For this review, take the finished solid that the model builds, in its own axes (mm). A direction names the side the tool comes from. Give positions to 0.01 mm unless a question says otherwise; leave off trailing zeros. Order: outer loops, then holes, each group sorted by start corner. A loop starts at its lowest first (then second) coordinate and runs counter-clockwise, first axis right, second up. Notation, with made-up numbers: M 65,36.25 L 75,36.25 A24 ccw 75,57.25 Z; hole C 82.25,70.5 d8. An arc over 180 degrees is marked long. Use CSV: the item, a comma, the result in double quotes. Start each with the question number.
(1) Consider section A-A (y = 15.5). Write out the cut boundary in (x, z), and give its area (3 significant figures).
(2) Consider section C-C (z = 10). Write out the cut boundary in (x, y), and give its area (3 significant figures).
(3) Tool access review of faces 1 (the face through (24.944, 46.744, 11.902)), 2 (the face through (7.56, 8.028, 13.062)), 3 (the face through (21, 26, 12)): name each direction out of +Z, -Z, +X, -X, +Y, -Y from which nothing blocks a thin tool from reaching the whole face with its end or side.
(4) Consider section B-B (x = 0). Write out the cut boundary in (y, z).
(5) Consider section D-D (y = 30). Write out the cut boundary in (x, z), and give its area (3 significant figures).
(6) Draft analysis for pull direction Y (two halves, no side actions). For faces 4 (the face through (5, 6, 7)), 5 (the face through (-8.44, 8.028, 13.062)), 6 (the face through (-24.944, 42.214, 12.553)), state which applies: pulls with the +Y half, pulls with the -Y half, needs draft (parallel to the pull), parting line crosses it, or undercut.
(7) Wall thickness on L1, parallel to Y at x = -25.75, z = 12; L2, parallel to X at y = 36, z = 2.5; L3, parallel to X at y = 8.5, z = 17: over which ranges is each line inside the solid? List them lowest first. Write a range as from..to.
(8) Clearance check with flat-ended pins moving along their axes: P1, Ø1.7, axis at y = 38, z = 20, coming from the +X side; P2, Ø1.2, axis at x = 5, z = 6, coming from the +Y side; P3, Ø1.1, axis at x = 6, z = 18, coming from the +Y side. State where each tip first meets the part, or that it passes through.
```python
from build123d import *

# Parameters (mm, degrees)
DODANIE_WYCI_GNI_CIE1_DEPTH = 24
SZKIC2_R                    = 4.25
WYTNIJ_WYCI_GNI_CIE1_DEPTH  = 81.249610591
SZKIC3_R                    = 0.65
SZKIC3_R_2                  = 4.25
WYTNIJ_WYCI_GNI_CIE2_DEPTH  = 55.927224579
SZKIC4_R                    = 0.75
WYTNIJ_WYCI_GNI_CIE3_DEPTH  = 81.249610591
SZKIC3_3_R                  = 1.15
SZKIC3_3_R_2                = 0.65
WYTNIJ_WYCI_GNI_CIE4_DEPTH  = 4


with BuildPart() as part:
    # Szkic1 → Dodanie-wyci_gni_cie1 (new body)
    with BuildSketch(Plane.XY):
        Polygon((21, 10), (-21, 10), (-21, 50), (-29, 50), (-29, 0), (29, 0), (29, 50), (21, 50), align=None)
    extrude(amount=DODANIE_WYCI_GNI_CIE1_DEPTH)

    # Szkic2 → Wytnij-wyci_gni_cie1 (cut, through all)
    with BuildSketch(Plane(origin=(29, 0, 0), x_dir=(0, 0, -1), z_dir=(1, 0, 0))):
        with BuildLine():
            ThreePointArc((-12, 50), (-3.514718626, 46.485281374), (0, 38))
            Line((0, 38), (0, 50))
            Line((0, 50), (-12, 50))
        make_face()
        with BuildLine():
            ThreePointArc((-24, 38), (-20.485281374, 46.485281374), (-12, 50))
            Line((-12, 50), (-24, 50))
            Line((-24, 50), (-24, 38))
        make_face()
        with Locations((-12, 38)):
            Circle(SZKIC2_R)
    extrude(amount=-WYTNIJ_WYCI_GNI_CIE1_DEPTH, mode=Mode.SUBTRACT)

    # Szkic3 → Wytnij-wyci_gni_cie2 (cut, through all)
    with BuildSketch(Plane(origin=(0, 10, 0), x_dir=(1, 0, 0), z_dir=(0, 1, 0))):
        with Locations(Location((0, -4, 0), (0, 0, 270))):
            Circle(SZKIC3_R)
        with Locations(Location((-5.656854249, -6.343145751, 0), (0, 0, 270))):
            Circle(SZKIC3_R)
        with Locations(Location((-8, -12, 0), (0, 0, 270))):
            Circle(SZKIC3_R)
        with Locations(Location((-5.656854249, -17.656854249, 0), (0, 0, 270))):
            Circle(SZKIC3_R)
        with Locations(Location((0, -20, 0), (0, 0, 270))):
            Circle(SZKIC3_R)
        with Locations(Location((5.656854249, -17.656854249, 0), (0, 0, 270))):
            Circle(SZKIC3_R)
        with Locations(Location((0, -12, 0), (0, 0, 270))):
            Circle(SZKIC3_R_2)
        with Locations(Location((8, -12, 0), (0, 0, 270))):
            Circle(SZKIC3_R)
        with Locations(Location((5.656854249, -6.343145751, 0), (0, 0, 270))):
            Circle(SZKIC3_R)
    extrude(amount=-WYTNIJ_WYCI_GNI_CIE2_DEPTH, mode=Mode.SUBTRACT)

    # Szkic4 → Wytnij-wyci_gni_cie3 (cut, through all)
    with BuildSketch(Plane.ZY.offset(29)):
        with Locations((12, 46)):
            Circle(SZKIC4_R)
        with Locations((17.656854249, 43.656854249)):
            Circle(SZKIC4_R)
        with BuildLine():
            ThreePointArc((3.25, 38), (4, 37.25), (4.75, 38))
            Line((4.75, 38), (3.25, 38))
        make_face()
        with BuildLine():
            Line((3.25, 38), (4.75, 38))
            ThreePointArc((4.75, 38), (4, 38.75), (3.25, 38))
        make_face()
        with Locations((6.343145751, 32.343145751)):
            Circle(SZKIC4_R)
        with Locations((17.656854249, 32.343145751)):
            Circle(SZKIC4_R)
        with Locations((20, 38)):
            Circle(SZKIC4_R)
        with Locations((12, 30)):
            Circle(SZKIC4_R)
        with Locations((6.343145751, 43.656854249)):
            Circle(SZKIC4_R)
    extrude(amount=-WYTNIJ_WYCI_GNI_CIE3_DEPTH, mode=Mode.SUBTRACT)

    # Szkic3_3 → Wytnij-wyci_gni_cie4 (cut)
    with BuildSketch(Plane(origin=(0, 10, 0), x_dir=(1, 0, 0), z_dir=(0, 1, 0))):
        with Locations(Location((8, -12, 0), (0, 0, 270))):
            Circle(SZKIC3_3_R)
        with Locations(Location((8, -12, 0), (0, 0, 270))):
            Circle(SZKIC3_3_R_2, mode=Mode.SUBTRACT)
        with Locations(Location((5.656854249, -6.343145751, 0), (0, 0, 270))):
            Circle(SZKIC3_3_R)
        with Locations(Location((5.656854249, -6.343145751, 0), (0, 0, 270))):
            Circle(SZKIC3_3_R_2, mode=Mode.SUBTRACT)
        with Locations(Location((0, -4, 0), (0, 0, 270))):
            Circle(SZKIC3_3_R)
        with Locations(Location((0, -4, 0), (0, 0, 270))):
            Circle(SZKIC3_3_R_2, mode=Mode.SUBTRACT)
        with Locations(Location((-5.656854249, -6.343145751, 0), (0, 0, 270))):
            Circle(SZKIC3_3_R)
        with Locations(Location((-5.656854249, -6.343145751, 0), (0, 0, 270))):
            Circle(SZKIC3_3_R_2, mode=Mode.SUBTRACT)
        with Locations(Location((-8, -12, 0), (0, 0, 270))):
            Circle(SZKIC3_3_R)
        with Locations(Location((-8, -12, 0), (0, 0, 270))):
            Circle(SZKIC3_3_R_2, mode=Mode.SUBTRACT)
        with Locations(Location((-5.656854249, -17.656854249, 0), (0, 0, 270))):
            Circle(SZKIC3_3_R)
        with Locations(Location((-5.656854249, -17.656854249, 0), (0, 0, 270))):
            Circle(SZKIC3_3_R_2, mode=Mode.SUBTRACT)
        with Locations(Location((0, -20, 0), (0, 0, 270))):
            Circle(SZKIC3_3_R)
        with Locations(Location((0, -20, 0), (0, 0, 270))):
            Circle(SZKIC3_3_R_2, mode=Mode.SUBTRACT)
        with Locations(Location((5.656854249, -17.656854249, 0), (0, 0, 270))):
            Circle(SZKIC3_3_R)
        with Locations(Location((5.656854249, -17.656854249, 0), (0, 0, 270))):
            Circle(SZKIC3_3_R_2, mode=Mode.SUBTRACT)
    extrude(amount=-WYTNIJ_WYCI_GNI_CIE4_DEPTH, mode=Mode.SUBTRACT)


solid = part.part
```
Check result:
1,outline,"M -29,0 L -21,0 L -21,24 L -29,24 Z; M 21,0 L 29,0 L 29,24 L 21,24 Z"
1,area,"384 mm^2"
2,outline,"M -29,0 L -3.75,0 L -3.75,10 L -21,10 L -21,34.25 L -29,34.25 Z; M -29,41.75 L -21,41.75 L -21,49.83 L -29,49.83 Z; M 3.75,0 L 29,0 L 29,34.25 L 21,34.25 L 21,10 L 3.75,10 Z; M 21,41.75 L 29,41.75 L 29,49.83 L 21,49.83 Z"
2,area,"1,020 mm^2"
3,face 1,"+X, -X"
3,face 2,"+Y"
3,face 3,"+Z, -Z, +Y"
4,outline,"M 0,0 L 10,0 L 10,2.85 L 6,2.85 L 6,3.35 L 0,3.35 Z; M 0,4.65 L 6,4.65 L 6,5.15 L 10,5.15 L 10,7.75 L 0,7.75 Z; M 0,16.25 L 10,16.25 L 10,18.85 L 6,18.85 L 6,19.35 L 0,19.35 Z; M 0,20.65 L 6,20.65 L 6,21.15 L 10,21.15 L 10,24 L 0,24 Z"
5,outline,"M -29,0 L -21,0 L -21,11.25 L -29,11.25 Z; M -29,12.75 L -21,12.75 L -21,24 L -29,24 Z; M 21,0 L 29,0 L 29,11.25 L 21,11.25 Z; M 21,12.75 L 29,12.75 L 29,24 L 21,24 Z"
5,area,"360 mm^2"
6,face 4,"pulls with the +Y half"
6,face 5,"needs draft"
6,face 6,"undercut"
7,L1,"y = 0..29.25, 30.75..33.75, 42.25..45.25, 46.75..50"
7,L2,"x = -29..-21, 21..29"
7,L3,"x = -29..-6.6, -4.71..4.71, 6.6..29"
8,P1,"stops at x = 29"
8,P2,"stops at y = 10"
8,P3,"stops at y = 6"
